Source: CAD feature listing. Evaluate the final solid. Frame: model axes, mm. Face numbers are marked on the shaded views. A direction names the side the tool comes from. Coordinates: 2 decimals unless noted, no trailing zeros. Loops run counter-clockwise (first coordinate to the right, second up) from the corner with the lowest first, then second, coordinate; pieces in that order, holes last.
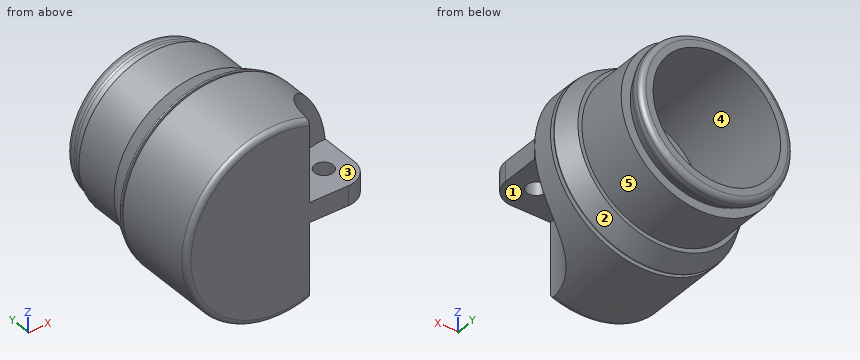
Autodesk Inventor part; units mm, degrees
ref_plane "Work Plane1" through (0, 10.3, 0) normal (0, 1, 0) x (1, 0, 0)
ref_plane "Work Plane2" through (0, 16.3, 0) normal (0, 1, 0) x (1, 0, 0)
ref_plane "Work Plane3" through (0, 0, 8.89) normal (0, 0, 1) x (1, 0, 0)
sketch "Sketch1" plane through (0, 0, 0) normal (0, 1, 0) x (-1, 0, 0)
  circle A0 centre (0, 0) radius 8.89
  dimension "d0" = 17.78
extrude "Extrusion1" add sketch "Sketch1" along normal blind 8
sketch "Sketch2" plane through (0, 8, 0) normal (0, 1, 0) x (1, 0, 0)
  circle A0 centre (0, 0) radius 7.62
  dimension "d3" = 15.24
extrude "Extrusion2" add sketch "Sketch2" along normal blind 0.3
ref_plane "Work Plane1" through (0, 10.3, 0) normal (0, 1, 0) x (1, 0, 0)
sketch "Sketch4" plane through (0, 10.3, 0) normal (0, 1, 0) x (1, 0, 0)
  circle A0 centre (0, 0) radius 8
  dimension "d7" = 16
sketch "Sketch5" plane through (0, 8.3, 0) normal (0, 1, 0) x (1, 0, 0)
  circle A0 centre (0, 0) radius 8.89
  dimension "d8" = 17.78
loft "Loft1" add profiles "Sketch5", "Sketch4"
sketch "Sketch6" plane through (0, 10.3, 0) normal (0, 1, 0) x (1, 0, 0)
  circle A0 centre (0, 0) radius 7.62
  dimension "d13" = 15.24
extrude "Extrusion3" add sketch "Sketch6" along normal blind 5
sketch "Sketch7" plane through (0, 15.3, 0) normal (0, 1, 0) x (1, 0, 0)
  circle A0 centre (0, 0) radius 6.75
  dimension "d16" = 13.5
ref_plane "Work Plane2" through (0, 16.3, 0) normal (0, 1, 0) x (1, 0, 0)
sketch "Sketch8" plane through (0, 16.3, 0) normal (0, 1, 0) x (1, 0, 0)
  circle A0 centre (0, 0) radius 7.25
  dimension "d18" = 14.5
loft "Loft2" add profiles "Sketch7", "Sketch8"
fillet "Fillet1" radius 0.08 1 edges at (-8.89, 8.3, 0)
thread "Thread1"
sketch "Sketch9" plane through (0, 16.3, 0) normal (0, 1, 0) x (1, 0, 0)
  circle A0 centre (0, 0) radius 7.25
extrude "Extrusion4" add sketch "Sketch9" along normal blind 1
ref_plane "Work Plane3" through (0, 0, 8.89) normal (0, 0, 1) x (1, 0, 0)
sketch "Sketch10" plane through (0, 0, 8.89) normal (0, 0, 1) x (1, 0, 0)
  line L0 (8.89, 0) -> (-8.89, 0)
  circle A0 centre (8.89, 0) radius 5.9795
  point P0 (0, 0)
extrude "Extrusion5" cut sketch "Sketch10" against normal blind 80
ref_plane "Work Plane4" through (8.89, 0, 0) normal (1, 0, 0) x (0, 1, 0)
sketch "Sketch11" plane through (8.89, 0, 0) normal (1, 0, 0) x (0, 1, 0)
  line L0 (0, -8.89) -> (0, 8.89)
  line L1 (5.9795, 0.6803) -> (0, 0.6803)
  line L2 (0, 0.6803) -> (0, -1.1889)
  line L3 (0, -1.1889) -> (5.9795, -1.1889)
  line L4 (5.9795, -1.1889) -> (5.9795, 0.6803)
  point P0 (0, 0)
  point P1 (0, -8.4001)
  point P2 (0, 8.4001)
extrude "Extrusion6" add sketch "Sketch11" against normal up to surface
sketch "Sketch12" plane through (8.89, 0, 0.6803) normal (0, 0, 1) x (1, 0, 0)
  circle A0 centre (-2.4423, 2.9044) radius 0.889
  point P0 (-8.89, 0)
  dimension "d34" = 1.778
extrude "Extrusion7" cut sketch "Sketch12" against normal blind 80
fillet "Fillet2" radius 2.286 1 edges at (8.89, 0, -0.2543)
fillet "Fillet3" radius 0.5 2 edges at (-5.1555, 0, 7.2424) (-5.1555, 0, -7.2424)
fillet "Fillet4" radius 0.5 1 edges at (-7.25, 16.3, 0)
fillet "Fillet5" radius 0.5 1 edges at (-7.25, 17.3, 0)
sketch "Sketch13" plane through (0, 17.3, 0) normal (0, 1, 0) x (1, 0, 0)
  circle A0 centre (0, 0) radius 6.0809
extrude "Extrusion8" cut sketch "Sketch13" against normal blind 10
properties part number "Tail Cap"
Q1. Reachability of the marked faces 1 and 2 from +Z, -Z, +X, -X, +Y, -Y: full face, straight path, thin tool, end or side. Return the list, or none.
Q2. Section query A-A on y = 12.5. Return the cut outline in (x, z).
Q3. First-contact query: pin 1 Ø4 at (x, y) = (-5.5, 10) entering from +Z; pin 2 Ø1 at (x, z) = (-6, -5) entering from +Y; pin 3 Ø5.5 at (x, z) = (3.5, -0.5) entering from -Y; pin 4 Ø1.5 at (y, z) = (2, -3.5) entering from +X. Flat tips, straight axial feed; report the tip coordinate or a pass-through.
Q4. Draft query along X for the marked faces 3, 4 and 5. Return one class per face: released by +X, released by -X, zero draft, split by the parting line, or undercut.
Q5. Section query B-B on y = 8.75. Return the cut outline in (x, z), then the cut area to 3 significant figures.
Q6. Material intervals for line 1 along Y through (x, z) = (0.5, -5.25); line 2 along Z through (x, y) = (0, 10.75); line 3 along Y through (x, z) = (4.75, -7), sorted ascending.
Resolved:
1. face 1: -Z, +X, -Y
1. face 2: +Y
2. outline: circle Ø15.24 at (0, 0); hole circle Ø12.16 at (0, 0)
3. pin 1: stops at z = 7.75
3. pin 2: stops at y = 15.3
3. pin 3: stops at y = 0
3. pin 4: stops at x = 3.58
4. face 3: zero draft
4. face 4: undercut
4. face 5: split by the parting line
5. outline: circle Ø17.38 at (0, 0); hole circle Ø12.16 at (0, 0)
5. area: 121 mm2
6. line 1: y = 0 to 7.3
6. line 2: z = -7.62 to -6.08, 6.08 to 7.62
6. line 3: y = 4.31 to 8, 8.3 to 9.27
